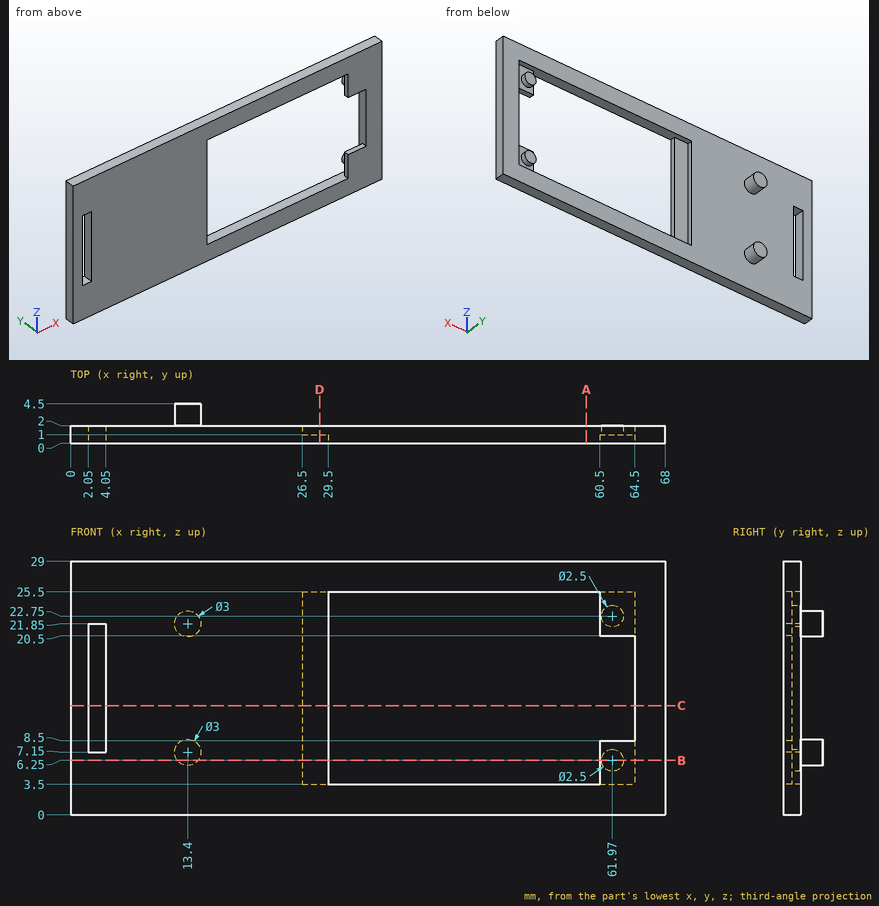
Source: three-view drawing plus pictorial views. Frame: mm from the lowest corner of the part. Give positions to 0.01 mm unless a question says otherwise; leave off trailing zeros. Order: outer loops, then holes, each group sorted by start corner. A loop starts at its lowest first (then second) coordinate and runs counter-clockwise, first axis right, second up. Notation, with made-up numbers: (41, 70.25) - (84, 70.25) arc R25 cw to (84, 103.25) - close; hole circle Ø6 at (60.25, 59.25). An arc over 180 degrees is marked (long way). Answer as a JSON object with one key per item and string values. Group by question number.
Q1. Cut plane D-D, the plane x = 28.5. Output: boundary loops of the cut face in (y, z).
Q2. Line query: probe 1 along X at (y, z) = (1.8, 9); probe 2 along Z at (x, y) = (51, 1.35); probe 3 along X at (y, z) = (0.25, 12.75). Output: solid intervals per line, ascending.
Q3. Cut plane A-A, the plane x = 59. Output: boundary loops of the cut face in (y, z).
Q4. Cut plane B-B, the plane z = 6.25. Output: boundary loops of the cut face in (x, y).
Q5. Cut plane C-C, the plane z = 12.5. Output: boundary loops of the cut face in (x, y).
Q6. First-contact query: pin 1 Ø1.2 at (x, z) = (62, 6) entering from +Y; pin 2 Ø2 at (x, y) = (17.5, 4) entering from +Z. Flat tips, straight axial feed; report the tip coordinate or a pass-through.
Results:
{
 "1": {"outline": "(0, 0) - (2, 0) - (2, 3.5) - (1, 3.5) - (1, 25.5) - (2, 25.5) - (2, 29) - (0, 29) - close"},
 "2": {"probe 1": "0 to 2.05, 4.05 to 26.5, 64.5 to 68", "probe 2": "0 to 3.5, 25.5 to 29", "probe 3": "0 to 2.05, 4.05 to 29.5, 64.5 to 68"},
 "3": {"outline": "(0, 0) - (2, 0) - (2, 3.5) - (0, 3.5) - close; (0, 25.5) - (2, 25.5) - (2, 29) - (0, 29) - close"},
 "4": {"outline": "(0, 0) - (29.5, 0) - (29.5, 1) - (26.5, 1) - (26.5, 2) - (14.6, 2) - (14.6, 4.5) - (12.2, 4.5) - (12.2, 2) - (0, 2) - close; (60.5, 0) - (68, 0) - (68, 2) - (64.5, 2) - (64.5, 1) - (63.22, 1) - (63.22, 2) - (60.72, 2) - (60.72, 1) - (60.5, 1) - close"},
 "5": {"outline": "(0, 0) - (2.05, 0) - (2.05, 2) - (0, 2) - close; (4.05, 0) - (29.5, 0) - (29.5, 1) - (26.5, 1) - (26.5, 2) - (4.05, 2) - close; (64.5, 0) - (68, 0) - (68, 2) - (64.5, 2) - close"},
 "6": {"pin 1": "y = 2", "pin 2": "through"}
}
